Check sheet for the modelled part. Datum: model origin and axes. Units: mm. Give positions to 0.01 mm unless a question says otherwise; leave off trailing zeros. Loops run counter-clockwise (first coordinate to the right, second up) from the corner with the lowest first, then second, coordinate; pieces in that order, holes last. Notation, with made-up numbers: (-8, -11.5) -> (39, -11.5) arc R18 cw to (39, 8.5) -> close; hole circle Ø1 at (-40, 31.25). An arc over 180 degrees is marked (long way). Write each question's results on one line, items separated by ' | '. Start each with the question number.
Item 1: Scan lines: line 1 along Y through (x, z) = (201.5, 1.45); line 2 along X through (y, z) = (-252.5, 0.35); line 3 along X through (y, z) = (32, 0.55). Record each from-to range of solid material in increasing order.
Item 2: Cross-section at B-B on y = 216.5. Enter the section's corners in (x, z) (3 decimals).
Item 3: Cross-section at A-A on x = -150. Enter the section's corners in (y, z) (3 decimals).
Item 4: Gauge pin test, flat ends, axial feed: pin 1 Ø1.6 at (x, z) = (-292.5, 1.5) entering from +Y; pin 2 Ø1 at (x, z) = (291.5, 1) entering from -Y; pin 3 Ø1.5 at (y, z) = (-110, 1) entering from -X. Record the tip position at first contact, or that the pin passes through.
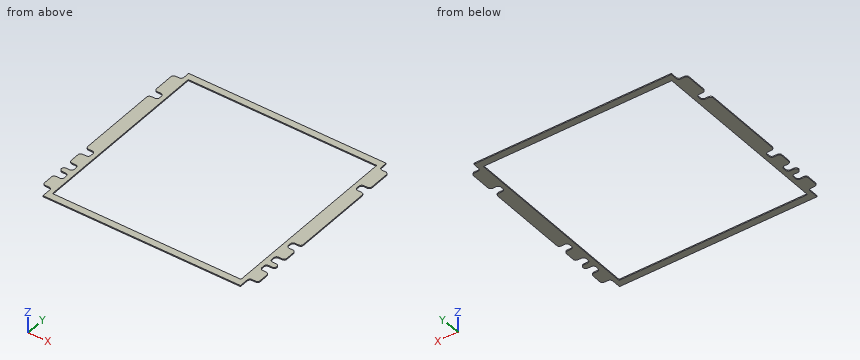
from build123d import *

# Parameters (mm, degrees)
SKETCH1_W           = 609.6
SKETCH1_H           = 559.70678
BOSS_EXTRUDE1_DEPTH = 3.175
SKETCH6_W           = 25.4
SKETCH6_H           = 33.599180378
SKETCH6_H_2         = 22.86
SKETCH6_H_3         = 26.284283972
CUT_EXTRUDE1_DEPTH  = 414.800725615
SKETCH7_W           = 533.4
SKETCH7_H           = 521.60678
CUT_EXTRUDE2_DEPTH  = 414.800725615
FILLET1_START       = -1
FILLET1_DEPTH       = 5
FILLET1_2_DEPTH     = 3.175


with BuildPart() as part:
    # Sketch1 → Boss-Extrude1 (new body)
    with BuildSketch(Plane.XY):
        Rectangle(SKETCH1_W, SKETCH1_H)
    extrude(amount=BOSS_EXTRUDE1_DEPTH)

    # Sketch6 → Cut-Extrude1 (cut, through all)
    with BuildSketch(Plane.XY.offset(3.175)):
        with Locations((292.1, -263.053799811)):
            Rectangle(SKETCH6_W, SKETCH6_H)
        with Locations((292.1, -193.67373)):
            Rectangle(SKETCH6_W, SKETCH6_H_2)
        with Locations((292.1, -155.57373)):
            Rectangle(SKETCH6_W, SKETCH6_H_2)
        with Locations((292.1, -92.07881)):
            Rectangle(SKETCH6_W, SKETCH6_H_2)
        with Locations((292.1, 171.90593)):
            Rectangle(SKETCH6_W, SKETCH6_H_2)
        with Locations((292.1, 266.711248014)):
            Rectangle(SKETCH6_W, SKETCH6_H_3)
    cut_extrude1 = extrude(amount=-CUT_EXTRUDE1_DEPTH, mode=Mode.SUBTRACT)

    # Sketch7 → Cut-Extrude2 (cut, through all)
    with BuildSketch(Plane.XY.offset(3.175)):
        Rectangle(SKETCH7_W, SKETCH7_H)
    extrude(amount=-CUT_EXTRUDE2_DEPTH, mode=Mode.SUBTRACT)

    # Mirror1: Cut-Extrude1 across plane
    add(cut_extrude1.mirror(Plane(origin=(0, 0, 0), x_dir=(0, 0, 1), z_dir=(1, 0, 0))), mode=Mode.SUBTRACT)

    # Fillet1: read off the stored shape, not the designer's step
    # Fillet1 outline → Fillet1 (cut)
    with BuildSketch(Plane.XY.offset(FILLET1_START)):
        with BuildLine():
            ThreePointArc((-297.18, -246.254209622), (-302.568153673, -244.022363295), (-304.8, -238.634209622))
            Line((-304.8, -238.634209622), (-304.8, -246.254209622))
            Line((-304.8, -246.254209622), (-297.18, -246.254209622))
        make_face()
        with BuildLine():
            ThreePointArc((-304.8, -212.72373), (-302.568153673, -207.335576327), (-297.18, -205.10373))
            Line((-297.18, -205.10373), (-304.8, -205.10373))
            Line((-304.8, -205.10373), (-304.8, -212.72373))
        make_face()
        with BuildLine():
            ThreePointArc((-297.18, -182.24373), (-302.568153673, -180.011883673), (-304.8, -174.62373))
            Line((-304.8, -174.62373), (-304.8, -182.24373))
            Line((-304.8, -182.24373), (-297.18, -182.24373))
        make_face()
        with BuildLine():
            ThreePointArc((-304.8, -174.62373), (-302.568153673, -169.235576327), (-297.18, -167.00373))
            Line((-297.18, -167.00373), (-304.8, -167.00373))
            Line((-304.8, -167.00373), (-304.8, -174.62373))
        make_face()
        with BuildLine():
            ThreePointArc((-297.18, -144.14373), (-302.568153673, -141.911883673), (-304.8, -136.52373))
            Line((-304.8, -136.52373), (-304.8, -144.14373))
            Line((-304.8, -144.14373), (-297.18, -144.14373))
        make_face()
        with BuildLine():
            ThreePointArc((-304.8, -111.12881), (-302.568153673, -105.740656327), (-297.18, -103.50881))
            Line((-297.18, -103.50881), (-304.8, -103.50881))
            Line((-304.8, -103.50881), (-304.8, -111.12881))
        make_face()
        with BuildLine():
            ThreePointArc((-297.18, -80.64881), (-302.568153673, -78.416963673), (-304.8, -73.02881))
            Line((-304.8, -73.02881), (-304.8, -80.64881))
            Line((-304.8, -80.64881), (-297.18, -80.64881))
        make_face()
        with BuildLine():
            ThreePointArc((-304.8, 152.85593), (-302.568153673, 158.244083673), (-297.18, 160.47593))
            Line((-297.18, 160.47593), (-304.8, 160.47593))
            Line((-304.8, 160.47593), (-304.8, 152.85593))
        make_face()
        with BuildLine():
            ThreePointArc((-297.18, 183.33593), (-302.568153673, 185.567776327), (-304.8, 190.95593))
            Line((-304.8, 190.95593), (-304.8, 183.33593))
            Line((-304.8, 183.33593), (-297.18, 183.33593))
        make_face()
        with BuildLine():
            ThreePointArc((-304.8, 245.949106028), (-302.568153672, 251.3372597), (-297.18, 253.569106028))
            Line((-297.18, 253.569106028), (-304.8, 253.569106028))
            Line((-304.8, 253.569106028), (-304.8, 245.949106028))
        make_face()
        with BuildLine():
            ThreePointArc((297.18, 253.569106028), (302.568153672, 251.3372597), (304.8, 245.949106028))
            Line((304.8, 245.949106028), (304.8, 253.569106028))
            Line((304.8, 253.569106028), (297.18, 253.569106028))
        make_face()
        with BuildLine():
            ThreePointArc((304.8, 190.95593), (302.568153673, 185.567776327), (297.18, 183.33593))
            Line((297.18, 183.33593), (304.8, 183.33593))
            Line((304.8, 183.33593), (304.8, 190.95593))
        make_face()
        with BuildLine():
            ThreePointArc((297.18, 160.47593), (302.568153673, 158.244083673), (304.8, 152.85593))
            Line((304.8, 152.85593), (304.8, 160.47593))
            Line((304.8, 160.47593), (297.18, 160.47593))
        make_face()
        with BuildLine():
            ThreePointArc((304.8, -73.02881), (302.568153673, -78.416963673), (297.18, -80.64881))
            Line((297.18, -80.64881), (304.8, -80.64881))
            Line((304.8, -80.64881), (304.8, -73.02881))
        make_face()
        with BuildLine():
            ThreePointArc((297.18, -103.50881), (302.568153673, -105.740656327), (304.8, -111.12881))
            Line((304.8, -111.12881), (304.8, -103.50881))
            Line((304.8, -103.50881), (297.18, -103.50881))
        make_face()
        with BuildLine():
            ThreePointArc((304.8, -136.52373), (302.568153673, -141.911883673), (297.18, -144.14373))
            Line((297.18, -144.14373), (304.8, -144.14373))
            Line((304.8, -144.14373), (304.8, -136.52373))
        make_face()
        with BuildLine():
            ThreePointArc((297.18, -167.00373), (302.568153673, -169.235576327), (304.8, -174.62373))
            Line((304.8, -174.62373), (304.8, -167.00373))
            Line((304.8, -167.00373), (297.18, -167.00373))
        make_face()
        with BuildLine():
            ThreePointArc((304.8, -174.62373), (302.568153673, -180.011883673), (297.18, -182.24373))
            Line((297.18, -182.24373), (304.8, -182.24373))
            Line((304.8, -182.24373), (304.8, -174.62373))
        make_face()
        with BuildLine():
            ThreePointArc((297.18, -205.10373), (302.568153673, -207.335576327), (304.8, -212.72373))
            Line((304.8, -212.72373), (304.8, -205.10373))
            Line((304.8, -205.10373), (297.18, -205.10373))
        make_face()
        with BuildLine():
            ThreePointArc((304.8, -238.634209622), (302.568153673, -244.022363295), (297.18, -246.254209622))
            Line((297.18, -246.254209622), (304.8, -246.254209622))
            Line((304.8, -246.254209622), (304.8, -238.634209622))
        make_face()
    extrude(amount=FILLET1_DEPTH, mode=Mode.SUBTRACT)

    # Fillet1 2 outline → Fillet1 2 (add)
    with BuildSketch(Plane.XY):
        with BuildLine():
            Line((-279.4, 253.569106028), (-279.4, 261.189106028))
            ThreePointArc((-279.4, 261.189106028), (-281.631846327, 255.800952355), (-287.02, 253.569106028))
            Line((-287.02, 253.569106028), (-279.4, 253.569106028))
        make_face()
        with BuildLine():
            Line((-279.4, -246.254209622), (-287.02, -246.254209622))
            ThreePointArc((-287.02, -246.254209622), (-281.631846327, -248.48605595), (-279.4, -253.874209622))
            Line((-279.4, -253.874209622), (-279.4, -246.254209622))
        make_face()
        with BuildLine():
            Line((-279.4, -205.10373), (-279.4, -197.48373))
            ThreePointArc((-279.4, -197.48373), (-281.631846327, -202.871883673), (-287.02, -205.10373))
            Line((-287.02, -205.10373), (-279.4, -205.10373))
        make_face()
        with BuildLine():
            Line((-279.4, -182.24373), (-287.02, -182.24373))
            ThreePointArc((-287.02, -182.24373), (-281.631846327, -184.475576327), (-279.4, -189.86373))
            Line((-279.4, -189.86373), (-279.4, -182.24373))
        make_face()
        with BuildLine():
            Line((-279.4, -167.00373), (-279.4, -159.38373))
            ThreePointArc((-279.4, -159.38373), (-281.631846327, -164.771883673), (-287.02, -167.00373))
            Line((-287.02, -167.00373), (-279.4, -167.00373))
        make_face()
        with BuildLine():
            Line((-279.4, -144.14373), (-287.02, -144.14373))
            ThreePointArc((-287.02, -144.14373), (-281.631846327, -146.375576327), (-279.4, -151.76373))
            Line((-279.4, -151.76373), (-279.4, -144.14373))
        make_face()
        with BuildLine():
            Line((-279.4, -103.50881), (-279.4, -95.88881))
            ThreePointArc((-279.4, -95.88881), (-281.631846327, -101.276963673), (-287.02, -103.50881))
            Line((-287.02, -103.50881), (-279.4, -103.50881))
        make_face()
        with BuildLine():
            Line((-279.4, -80.64881), (-287.02, -80.64881))
            ThreePointArc((-287.02, -80.64881), (-281.631846327, -82.880656327), (-279.4, -88.26881))
            Line((-279.4, -88.26881), (-279.4, -80.64881))
        make_face()
        with BuildLine():
            Line((-279.4, 160.47593), (-279.4, 168.09593))
            ThreePointArc((-279.4, 168.09593), (-281.631846327, 162.707776327), (-287.02, 160.47593))
            Line((-287.02, 160.47593), (-279.4, 160.47593))
        make_face()
        with BuildLine():
            Line((-279.4, 183.33593), (-287.02, 183.33593))
            ThreePointArc((-287.02, 183.33593), (-281.631846327, 181.104083673), (-279.4, 175.71593))
            Line((-279.4, 175.71593), (-279.4, 183.33593))
        make_face()
        with BuildLine():
            Line((279.4, -246.254209622), (279.4, -253.874209622))
            ThreePointArc((279.4, -253.874209622), (281.631846327, -248.48605595), (287.02, -246.254209622))
            Line((287.02, -246.254209622), (279.4, -246.254209622))
        make_face()
        with BuildLine():
            Line((279.4, 253.569106028), (287.02, 253.569106028))
            ThreePointArc((287.02, 253.569106028), (281.631846327, 255.800952355), (279.4, 261.189106028))
            Line((279.4, 261.189106028), (279.4, 253.569106028))
        make_face()
        with BuildLine():
            Line((279.4, 183.33593), (279.4, 175.71593))
            ThreePointArc((279.4, 175.71593), (281.631846327, 181.104083673), (287.02, 183.33593))
            Line((287.02, 183.33593), (279.4, 183.33593))
        make_face()
        with BuildLine():
            Line((279.4, 160.47593), (287.02, 160.47593))
            ThreePointArc((287.02, 160.47593), (281.631846327, 162.707776327), (279.4, 168.09593))
            Line((279.4, 168.09593), (279.4, 160.47593))
        make_face()
        with BuildLine():
            Line((279.4, -80.64881), (279.4, -88.26881))
            ThreePointArc((279.4, -88.26881), (281.631846327, -82.880656327), (287.02, -80.64881))
            Line((287.02, -80.64881), (279.4, -80.64881))
        make_face()
        with BuildLine():
            Line((279.4, -103.50881), (287.02, -103.50881))
            ThreePointArc((287.02, -103.50881), (281.631846327, -101.276963673), (279.4, -95.88881))
            Line((279.4, -95.88881), (279.4, -103.50881))
        make_face()
        with BuildLine():
            Line((279.4, -144.14373), (279.4, -151.76373))
            ThreePointArc((279.4, -151.76373), (281.631846327, -146.375576327), (287.02, -144.14373))
            Line((287.02, -144.14373), (279.4, -144.14373))
        make_face()
        with BuildLine():
            Line((279.4, -167.00373), (287.02, -167.00373))
            ThreePointArc((287.02, -167.00373), (281.631846327, -164.771883673), (279.4, -159.38373))
            Line((279.4, -159.38373), (279.4, -167.00373))
        make_face()
        with BuildLine():
            Line((279.4, -182.24373), (279.4, -189.86373))
            ThreePointArc((279.4, -189.86373), (281.631846327, -184.475576327), (287.02, -182.24373))
            Line((287.02, -182.24373), (279.4, -182.24373))
        make_face()
        with BuildLine():
            Line((279.4, -205.10373), (287.02, -205.10373))
            ThreePointArc((287.02, -205.10373), (281.631846327, -202.871883673), (279.4, -197.48373))
            Line((279.4, -197.48373), (279.4, -205.10373))
        make_face()
    extrude(amount=FILLET1_2_DEPTH)


solid = part.part
Answer sheet:
1) line 1: y = -279.85 to -260.8, 260.8 to 279.85 | line 2: x = -279.52 to -266.7, 266.7 to 279.52 | line 3: x = -304.8 to -266.7, 266.7 to 304.8
2) outline: (-304.8, 0) -> (-266.7, 0) -> (-266.7, 3.175) -> (-304.8, 3.175) -> close; (266.7, 0) -> (304.8, 0) -> (304.8, 3.175) -> (266.7, 3.175) -> close
3) outline: (-279.853, 0) -> (-260.803, 0) -> (-260.803, 3.175) -> (-279.853, 3.175) -> close; (260.803, 0) -> (279.853, 0) -> (279.853, 3.175) -> (260.803, 3.175) -> close
4) pin 1: stops at y = 253.57 | pin 2: stops at y = -246.25 | pin 3: stops at x = -304.79
